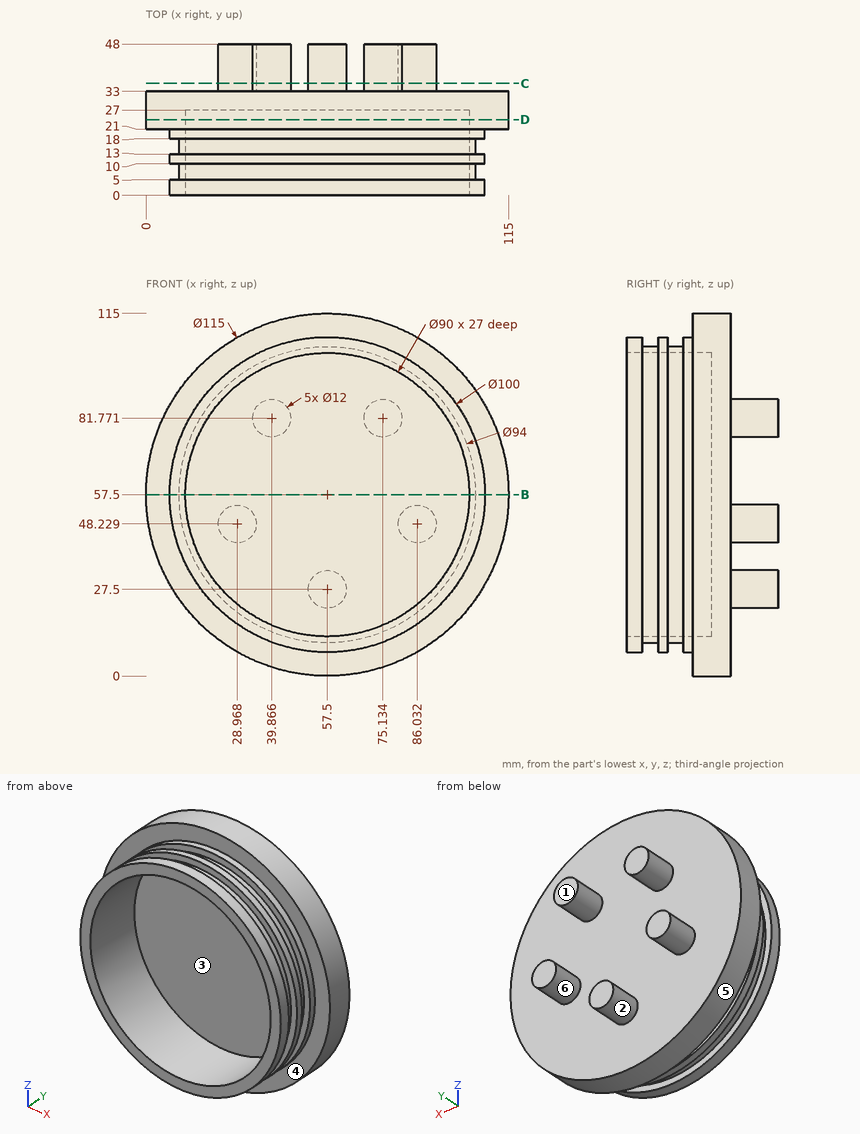
Here's the drawing with two shaded views (mm, measured from the low corner). I have some questions. A direction names the side the tool comes from. Round coordinates to 2 decimals unless told otherwise and drop trailing zeros. Loops run counter-clockwise (first coordinate to the right, second up) from the corner with the lowest first, then second, coordinate; pieces in that order, holes last. Notation, with made-up numbers: M 38,67.5 L 46,67.5 A31 cw 46,102.5 Z; hole C 64,28 d7. An arc over 180 degrees is marked long. Answer as a JSON object with one key per item and string values. Group by question number.
Q1. Imagine slicing it at B-B, the plane z = 57.5. Please give me the cut outline in (x, y).
Q2. Will these pins go through, and if not, where does the flat tip stop? pin 1 (5 mm diameter, centred on x = 54.5, y = 16.5, fed in from -Z); pin 2 (6 mm diameter, centred on x = 81, y = 7, fed in from -Z); pin 3 (4 mm diameter, centred on x = 95, y = 41, fed in from +Z); pin 4 (1 mm diameter, centred on x = 52, y = 34.5, fed in from -Z) (1 decimal).
Q3. Imagine slicing it at D-D, the plane y = 24. Please give me the cut outline in (x, z).
Q4. Imagine slicing it at C-C, the plane y = 35.5. Please give me the cut outline in (x, z).
Q5. We'd pull the mould along X, two halves only. Please class the marked faces 4, 5 and 6: +X half, -X half, draft (parallel to the pull), parting line (faces both ways), or undercut.
Q6. Please list where these lines run through material, in increasing order: L1, parallel to Y at x = 97, z = 29; L2, parallel to X at y = 8.75, z = 57.5; L3, parallel to X at y = 19.75, z = 57.5.
Q7. On a 3-axis mill with a long thin cutter (end or side, diameter ignored), from which of +Z, -Z, +X, -X, +Y, -Y can I reach the whole of each face in a straight line? I mean the marked faces 1, 2 and 3. Say none if no direction works.
Findings:
{
 "1": {"outline": "M 0,21 L 7.5,21 L 7.5,18 L 10.5,18 L 10.5,13 L 7.5,13 L 7.5,10 L 10.5,10 L 10.5,5 L 7.5,5 L 7.5,0 L 12.5,0 L 12.5,27 L 102.5,27 L 102.5,0 L 107.5,0 L 107.5,5 L 104.5,5 L 104.5,10 L 107.5,10 L 107.5,13 L 104.5,13 L 104.5,18 L 107.5,18 L 107.5,21 L 115,21 L 115,33 L 0,33 Z"},
 "2": {"pin 1": "stops at z = 7.51", "pin 2": "stops at z = 12.25", "pin 3": "passes through", "pin 4": "stops at z = 24.2"},
 "3": {"outline": "C 57.5,57.5 d115; hole C 57.5,57.5 d90"},
 "4": {"outline": "C 28.97,48.23 d12; C 39.87,81.77 d12; C 57.5,27.5 d12; C 75.13,81.77 d12; C 86.03,48.23 d12"},
 "5": {"face 4": "draft", "face 5": "parting line", "face 6": "undercut"},
 "6": {"L1": "y = 0 to 5, 10 to 13, 18 to 33", "L2": "x = 10.5 to 12.5, 102.5 to 104.5", "L3": "x = 7.5 to 12.5, 102.5 to 107.5"},
 "7": {"face 1": "+Z, -Z, +X, -X, +Y", "face 2": "+Y", "face 3": "-Y"}
}
